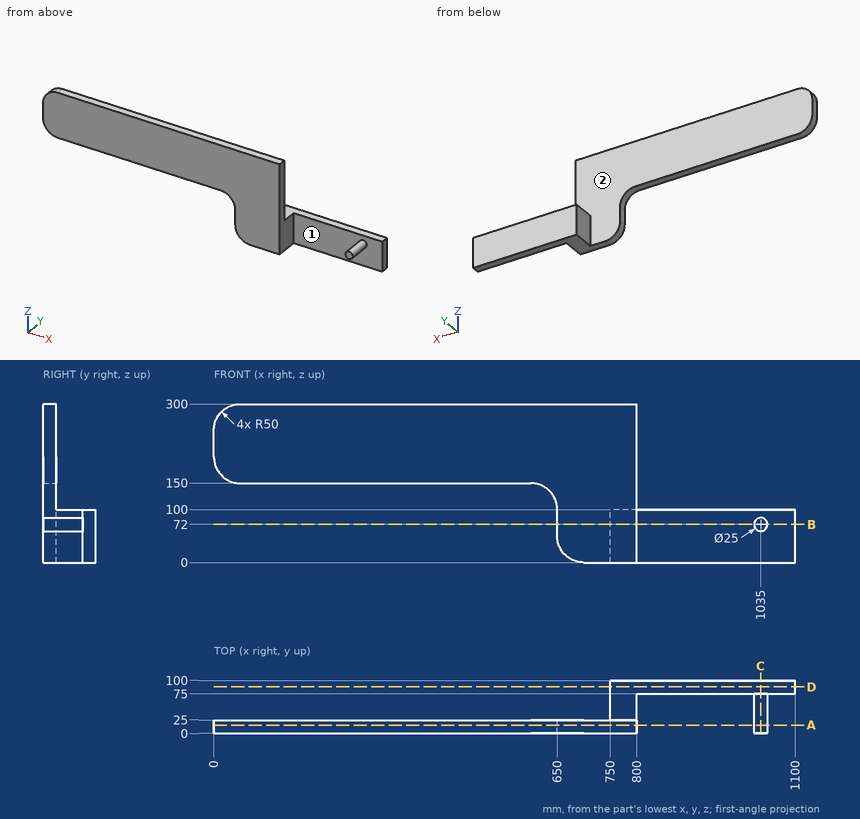
Here's the drawing with two shaded views (mm, measured from the low corner). I have some questions. Round coordinates to 2 decimals unless told otherwise and drop trailing zeros. Write each loop counter-clockwise with the first axis right and the second up, starting at its lowest first coordinate (ties: lowest second). Pieces come first, ordered by that corner, then holes. Notation, with made-up numbers: M 23.25,23 L 36.25,23 A11 cw 36.25,44 Z; hole C 1,-34 d2. An arc over 180 degrees is marked long. Use CSV: the item, a comma, the result in double quotes.
(1) Imagine slicing it at D-D (y = 88). Write out the boundary of the cut face in (x, z), plus the area to 3 significant figures.
Check values:
outline,"M 750,0 L 1100,0 L 1100,100 L 750,100 Z"
area,"35,000 mm^2"
(2) We'd pull the mould along X, two halves only. Please class the marked faces 1 and 2: +X half, -X half, draft (parallel to the pull), parting line (faces both ways), or undercut.
Check values:
face 1,"undercut"
face 2,"draft"
(3) Imagine slicing it at C-C (x = 1035). Write out the boundary of the cut face in (y, z).
Check values:
outline,"M 0,59.5 L 75,59.5 L 75,0 L 100,0 L 100,100 L 75,100 L 75,84.5 L 0,84.5 Z"
(4) I need wall thicknesses on line 1 along Y through (x, z) = (743, 97); line 2 along X through (y, z) = (60, 22.5); line 3 along X through (y, z) = (90.5, 59.5). Which ranges of each line are inside material? Lowest first, please.
Check values:
line 1,"0 to 25"
line 2,"750 to 800"
line 3,"750 to 1100"
(5) I'm going to push flat-ended pins straight in: pin 1 (12.5 mm diameter, centred on x = 244.5, y = 7.5, fed in from -Z); pin 2 (3 mm diameter, centred on y = 12.5, z = 120, fed in from -X); pin 3 (7.5 mm diameter, centred on y = 16, z = 86.5, fed in from -X). Where does each tip first touch, or does it pass through?
Check values:
pin 1,"z = 150"
pin 2,"x = 645.14"
pin 3,"x = 650"
(6) Imagine slicing it at A-A (y = 15.5). Write out the boundary of the cut face in (x, z), plus the area to 3 significant figures.
Check values:
outline,"M 0,200 A50 ccw 50,150 L 600,150 A50 cw 650,100 L 650,50 A50 ccw 700,0 L 800,0 L 800,300 L 50,300 A50 ccw 0,250 Z; C 1035,72 d25"
area,"142,000 mm^2"
(7) Imagine slicing it at B-B (z = 72). Write out the boundary of the cut face in (x, y).
Check values:
outline,"M 650,0 L 800,0 L 800,75 L 1022.5,75 L 1022.5,0 L 1047.5,0 L 1047.5,75 L 1100,75 L 1100,100 L 750,100 L 750,25 L 650,25 Z"
